For this review, take the finished solid that the model builds, in its own axes (mm). Face numbers are marked on the shaded views. Give positions to 0.01 mm unless a question says otherwise; leave off trailing zeros. Order: outer loops, then holes, each group sorted by start corner. A loop starts at its lowest first (then second) coordinate and runs counter-clockwise, first axis right, second up. Notation, with made-up numbers: (18, 71.5) - (70, 71.5) arc R21 ccw to (70, 83.5) - close; hole circle Ø2 at (-40, -17). An arc over 180 degrees is marked (long way). Use a Markdown table: item, result. Add a question column.
1) Wall thickness on L1, parallel to Z at x = -31, y = 8; L2, parallel to Y at x = -12, z = 34; L3, parallel to Y at x = 31, z = 2: over which ranges is each line inside the solid? List them lowest first.
2) We need section B-B on x = -1.5. Write out the cut boundary in (y, z).
3) We need section A-A on y = -18. Write out the cut boundary in (x, z).
4) Clearance check with flat-ended pins moving along their axes: P1, Ø5, axis at x = -23.5, y = 22, coming from the +Z side; P2, Ø4, axis at y = 7.5, z = 25.5, coming from the +X side; P3, Ø3, axis at x = 20, y = 21, coming from the -Z side. State where each tip first meets the part, or that it passes through.
5) Mouldability with a two-part tool opening along Y and no side actions: class the marked faces 1, 2 and 3 as released by +Y, released by -Y, zero draft, split by the parting line, or undercut.
```python
from build123d import *

# Parameters (mm, degrees)
SKETCH1_W                = 85.03995341
SKETCH1_H                = 85.695176246
BOSS_EXTRUDE1_DEPTH      = 30
BOSS_EXTRUDE1_DEPTH_BACK = 30
FILLET1_R                = 30
FILLET2_R                = 20
FILLET3_R                = 10


with BuildPart() as part:
    # Sketch1 → Boss-Extrude1 (new body, two sides)
    with BuildSketch(Plane(origin=(0, 0, 0), x_dir=(1, 0, 0), z_dir=(0, 1, 0))) as boss_extrude1_sk:
        Rectangle(SKETCH1_W, SKETCH1_H)
    extrude(amount=BOSS_EXTRUDE1_DEPTH)
    extrude(boss_extrude1_sk.sketch, amount=-BOSS_EXTRUDE1_DEPTH_BACK)

    # Fillet1
    fillet1_edges = [part.edges().sort_by_distance(p)[0] for p in [
        (42.519976705, 0, 42.847588123),
        (-42.519976705, 0, 42.847588123),
        (-42.519976705, 0, -42.847588123),
        (42.519976705, 0, -42.847588123),
    ]]
    fillet(fillet1_edges, radius=FILLET1_R)

    # Fillet2
    fillet2_edges = [part.edges().sort_by_distance(p)[0] for p in [
        (0, 30, 42.847588123),
        (42.519976705, 30, 0),
        (0, 30, -42.847588123),
        (-42.519976705, 30, 0),
        (-33.73318014, 30, -34.060791558),
        (-33.73318014, 30, 34.060791558),
        (33.73318014, 30, -34.060791558),
        (33.73318014, 30, 34.060791558),
    ]]
    fillet(fillet2_edges, radius=FILLET2_R)

    # Fillet3
    fillet3_edges = [part.edges().sort_by_distance(p)[0] for p in [
        (0, -30, 42.847588123),
        (42.519976705, -30, 0),
        (-42.519976705, -30, 0),
        (0, -30, -42.847588123),
        (-33.73318014, -30, -34.060791558),
        (-33.73318014, -30, 34.060791558),
        (33.73318014, -30, -34.060791558),
        (33.73318014, -30, 34.060791558),
    ]]
    fillet(fillet3_edges, radius=FILLET3_R)


solid = part.part
```
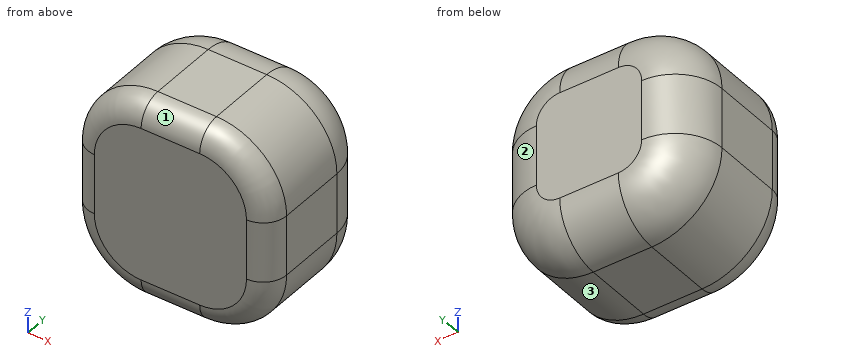
Checked values:
| question | item | result |
|---|---|---|
| 1 | L1 | -36.48 to 36.48 |
| 1 | L2 | -29.93 to 26.6 |
| 1 | L3 | -30 to 28.11 |
| 2 | outline | (-30, -32.85) arc R10 ccw to (-20, -42.85) - (10, -42.85) arc R20 ccw to (30, -22.85) - (30, 22.85) arc R20 ccw to (10, 42.85) - (-20, 42.85) arc R10 ccw to (-30, 32.85) - close |
| 3 | outline | (-42.52, -12.85) arc R30 ccw to (-12.52, -42.85) - (12.52, -42.85) arc R30 ccw to (42.52, -12.85) - (42.52, 12.85) arc R30 ccw to (12.52, 42.85) - (-12.52, 42.85) arc R30 ccw to (-42.52, 12.85) - close |
| 4 | P1 | z = 38.48 |
| 4 | P2 | x = 40.57 |
| 4 | P3 | z = -39.51 |
| 5 | face 1 | released by -Y |
| 5 | face 2 | released by +Y |
| 5 | face 3 | zero draft |
